```python
from build123d import *

# Parameters (mm, degrees)
F0_W     = 37
F0_H     = 3
F1_DEPTH = 15
F6_D     = 4.5
F7_D     = 4.5
F5_R     = 10


with BuildPart() as f1:
    # F0 (on Top) → F1 (new body)
    with BuildSketch(Plane.XY):
        Polygon((-23.234105, 31.848193), (-26.234105, 31.848193), (-26.234105, -8.151807), (-23.234105, -8.151807), (-23.234105, -5.151807), align=None)
        with Locations((-4.734105, -6.651807)):
            Rectangle(F0_W, F0_H)
    extrude(amount=F1_DEPTH)

    # F6 (through all)
    with Locations(Plane(origin=(-26.234105, 0, 0), x_dir=(0, -1, 0), z_dir=(-1, 0, 0))):
        with Locations((-24.348193, 7.5)):
            Hole(F6_D / 2)

    # F7 (through all)
    with Locations(Plane.XZ.offset(8.151807)):
        with Locations((6.265895, 7.5)):
            Hole(F7_D / 2)

    # F5
    f5_edges = [f1.edges().sort_by_distance(p)[0] for p in [
        (-23.234105, -5.151807, 7.5),
    ]]
    fillet(f5_edges, radius=F5_R)


solid = f1.part
```
Work out the finished part from the listing and answer in its coordinate system (mm). A direction names the side the tool comes from. Round coordinates to 2 decimals unless told otherwise and drop trailing zeros. Write each loop counter-clockwise with the first axis right and the second up, starting at its lowest first coordinate (ties: lowest second). Pieces come first, ordered by that corner, then holes. Notation, with made-up numbers: (-19.5, 89) -> (22.5, 89) arc R12 cw to (22.5, 102) -> close; hole circle Ø11 at (87, 82). An arc over 180 degrees is marked (long way). Write each question's results on one line, items separated by ' | '.
1) Which of the six approach directions +Z, -Z, +X, -X, +Y, -Y give full straight-line access (tool end or side, diameter ignored) to faces 1 (the flat face through (-7, -8.152, 7)), 2 (the flat face through (-23.234, 18, 7))?
Findings:
face 1: +Z, -Z, +X, -X, -Y | face 2: +Z, -Z, +X, +Y
2) Consider line 1 along Y through (x, z) = (-13, 1.5); line 2 along X through (y, z) = (8.5, 13.5); line 3 along Y through (x, z) = (-14, 8.25). Determine where each line is inside the solid, lowest interval first. Write a range as [from, to].
Findings:
line 1: y = [-8.15, -5.15] | line 2: x = [-26.23, -23.23] | line 3: y = [-8.15, -5.12]
3) For a pull along Z with two mould halves and no side action, classify faces 3 (the flat face through (-20, -3, 0)), 4 (the flat face through (13.766, -7, 7)), 5 (the cylindrical face through (-24.713, 25.558, 9.397)) as +Z half, -Z half, draft (parallel to the pull), parting line (faces both ways), or undercut.
Findings:
face 3: -Z half | face 4: draft | face 5: undercut
4) The part is cut by section D-D (y = 7). Write down the section's boundary in (x, z), and give its area (3 significant figures).
Findings:
outline: (-26.23, 0) -> (-23.23, 0) -> (-23.23, 15) -> (-26.23, 15) -> close | area: 45.0 mm²
5) Flat-ended cylindrical pins translate along their axes: pin 1 (6 mm diameter, centred on x = 6.27, z = 7.5, fed in from +Y); pin 2 (2.5 mm diameter, centred on y = 24.35, z = 7.5, fed in from -X); pin 3 (1 mm diameter, centred on y = 18.5, z = 7.5, fed in from +X). Find the tip coordinate at first contact, or state that the pin passes through.
Findings:
pin 1: stops at y = -5.15 | pin 2: passes through | pin 3: stops at x = -23.23
6) The part is cut by section C-C (z = 12). Write down the section's boundary in (x, y).
Findings:
outline: (-26.23, -8.15) -> (13.77, -8.15) -> (13.77, -5.15) -> (-13.23, -5.15) arc R10 cw to (-23.23, 4.85) -> (-23.23, 31.85) -> (-26.23, 31.85) -> close
7) The part is cut by section A-A (z = 7.5). Write down the section's boundary in (x, y), and give its area (3 significant figures).
Findings:
outline: (-26.23, -8.15) -> (4.02, -8.15) -> (4.02, -5.15) -> (-13.23, -5.15) arc R10 cw to (-23.23, 4.85) -> (-23.23, 22.1) -> (-26.23, 22.1) -> close; (-26.23, 26.6) -> (-23.23, 26.6) -> (-23.23, 31.85) -> (-26.23, 31.85) -> close; (8.52, -8.15) -> (13.77, -8.15) -> (13.77, -5.15) -> (8.52, -5.15) -> close | area: 225 mm²
8) The part is cut by section B-B (x = 5.5). Write down the section's boundary in (y, z).
Findings:
outline: (-8.15, 0) -> (-5.15, 0) -> (-5.15, 5.38) -> (-8.15, 5.38) -> close; (-8.15, 9.62) -> (-5.15, 9.62) -> (-5.15, 15) -> (-8.15, 15) -> close
